Build history of the part. All positions in model axes, mm. A direction names the side the tool comes from. Give positions to 0.01 mm unless a question says otherwise; leave off trailing zeros. Order: outer loops, then holes, each group sorted by start corner. A loop starts at its lowest first (then second) coordinate and runs counter-clockwise, first axis right, second up. Notation, with made-up numbers: (-35, 81) - (19, 81) arc R11 cw to (19, 86) - close; hole circle Ø11 at (-39, 87.5). An arc over 180 degrees is marked (long way). Use a Markdown table: item, result. Add a question column.
(1) Slice it at A-A (z = 40). Write the cut outline in (x, y), then the cut area to 3 significant figures.
(2) Flat gauge pins, fed straight in: pin 1 (6 mm diameter, centred on x = -19, z = 55.5, fed in from -Y); pin 2 (9 mm diameter, centred on y = 9, z = 10, fed in from -X); pin 3 (0.6 mm diameter, centred on y = -11.5, z = 50, fed in from +X). Where does each tip first touch, or does it go through?
(3) Which spindle directions (+Z, -Z, +X, -X, +Y, -Y) get a long thin tool onto all of the face, cutting with end or side? Do faces 5 (the face through (-2.03, -33.32, 8.52)), 6 (the face through (-4, 11, 39)), 7 (the face through (-8, -22, 39)), 8 (the face through (-17, -26, 39)). Say none if no direction does.
(4) Slice it at B-B (z = 10). Write the cut outline in (x, y), then the cut area to 3 significant figures.
(5) Slice it at C-C (x = -14). Write the cut outline in (y, z), then the cut area to 3 significant figures.
(6) Wall check: line 1 (Y direction, x = -1.5, z = 70); line 2 (Z direction, x = -2.3, y = 9); line 3 (Z direction, x = -9, y = -24.9). Give the ranges that are in metal, low to high.
(7) Mould opens along Z. For faces 1 (the face through (-29, -11, 39)), 2 (the face through (-19, -22, 0)), 3 (the face through (-14, -24, 80)), 4 (the face through (-9.121, 2.028, 22.747)) say: +Z half, -Z half, draft (parallel to the pull), parting line (faces both ways), or undercut.
(8) Slice it at D-D (y = 9). Write the cut outline in (x, z).
Autodesk Inventor part; units mm, degrees
ref_plane "YZ Plane" through (0, 0, 0) normal (1, 0, 0) x (0, 1, 0)
ref_plane "XZ Plane" through (0, 0, 0) normal (0, 1, 0) x (-1, 0, 0)
ref_plane "XY Plane" through (0, 0, 0) normal (0, 0, 1) x (1, 0, 0)
sketch "Sketch1" plane through (0, 0, 0) normal (0, 0, 1) x (1, 0, 0)
  line L0 (0, 0) -> (-29, 0)
  line L1 (-29, 0) -> (-29, 4)
  line L2 (-29, 4) -> (-4, 4)
  line L3 (-4, 4) -> (-4, 18)
  line L4 (-4, 18) -> (0, 18)
  line L5 (0, 18) -> (0, 0)
  dimension "d0" = 4
  dimension "d1" = 4
  dimension "d2" = 29
  dimension "d3" = 18
extrude "Extrusion1" add sketch "Sketch1" along normal blind 80
sketch "Sketch3" plane through (0, 0, 0) normal (1, 0, 0) x (0, 0, -1)
  line L0 (0, 0) -> (-80, 0)
  line L1 (-80, 0) -> (-80, 18)
  line L2 (0, 0) -> (0, 18)
  point P0 (-70, 9)
  point P1 (-10, 9)
  dimension "d9" = 9
  dimension "d10" = 10
  dimension "d11" = 10
hole "Hole1" at (0, 9, 70) at (0, 9, 10) direction (-1, 0, 0) diameter 5.5 end through all
sketch "Sketch4" plane through (-29, 0, 0) normal (0, -1, 0) x (1, 0, 0)
  line L0 (29, 0) -> (29, 80)
  line L1 (0, 0) -> (29, 0)
  point P0 (20, 60)
  point P1 (20, 20)
  dimension "d19" = 9
  dimension "d20" = 20
  dimension "d21" = 20
hole "Hole2" at (-9, 0, 60) at (-9, 0, 20) direction (0, 1, 0) diameter 5.5 end through all
sketch "Sketch9" plane through (-29, 0, 0) normal (0, -1, 0) x (1, 0, 0)
  line L0 (25, 80) -> (0, 80)
  line L1 (25, 0) -> (0, 0)
  line L2 (0, 80) -> (3, 80)
  line L3 (3, 80) -> (3, 0)
  line L4 (3, 0) -> (0, 0)
  line L5 (0, 0) -> (0, 80)
  point P0 (29, 0)
  point P1 (3, 80)
  dimension "d57" = 3
extrude "Extrusion5" add sketch "Sketch9" along normal blind 26
sketch "Sketch10" plane through (-26, 0, 80) normal (1, 0, 0) x (0, 0, -1)
  line L0 (80, -26) -> (0, -26)
  line L1 (80, 4) -> (80, -26)
  line L2 (0, -26) -> (80, -26)
  line L3 (80, -26) -> (80, -22)
  line L4 (80, -22) -> (0, -22)
  line L5 (0, -22) -> (0, -26)
  point P0 (80, 0)
  dimension "d60" = 4
extrude "Extrusion6" add sketch "Sketch10" along normal blind 26
sketch "Sketch11" plane through (-29, -26, 0) normal (0, -1, 0) x (1, 0, 0)
  line L0 (29, 80) -> (25, 80)
  line L1 (25, 0) -> (0, 0)
  line L2 (29, 80) -> (25, 80)
  line L3 (25, 80) -> (25, 0)
  line L4 (25, 0) -> (29, 0)
  line L5 (29, 0) -> (29, 80)
  point P0 (29, 0)
  dimension "d63" = 4
extrude "Extrusion7" add sketch "Sketch11" along normal blind 14
sketch "Sketch12" plane through (0, 0, 80) normal (1, 0, 0) x (0, 0, -1)
  circle A0 centre (10, 9) radius 2.75
  circle A1 centre (70, 9) radius 2.75
  line L0 (80, 18) -> (0, 18)
  line L1 (80, -40) -> (0, -40)
  line L2 (80, -22) -> (0, -22)
  point P0 (80, 0)
  point P1 (10, -31)
  point P2 (70, -31)
  point P3 (51, 18)
  dimension "d66" = 9
  dimension "d85" = 9
hole "Hole5" at (0, -31, 70) at (0, -31, 10) direction (-1, 0, 0) diameter 5.5 end through all
sketch "Sketch14" plane through (-26, -22, 80) normal (0, 1, 0) x (1, 0, 0)
  circle A0 centre (17, 20) radius 2.75
  circle A1 centre (17, 60) radius 2.75
  point P0 (26, 80)
hole "Hole6" at (-9, -22, 60) at (-9, -22, 20) direction (0, -1, 0) diameter 5.5 end through all
sketch "Sketch24" plane through (0, 0, 80) normal (1, 0, 0) x (0, 0, -1)
  line L0 (80, -40) -> (0, -40)
  line L1 (0, -22) -> (0, -40)
  point P0 (80, 0)
  point P1 (40, -31.5)
  dimension "d157" = 8.5
  dimension "d158" = 40
hole "Hole9" at (0, -31.5, 40) direction (-1, 0, 0) diameter 4.5 depth 8 tip angle 118
fillet "Fillet1" radius 10 2 edges at (-26, -22, 40) (-26, 0, 40)
Solution:
| question | item | result |
|---|---|---|
| 1 | outline | (-29, -26) - (-4, -26) - (-4, -29.25) - (0, -29.25) - (0, -22) - (-16, -22) arc R10 cw to (-26, -12) - (-26, -10) arc R10 cw to (-16, 0) - (0, 0) - (0, 18) - (-4, 18) - (-4, 4) - (-29, 4) - close; (-4, -40) - (0, -40) - (0, -33.75) - (-4, -33.75) - close |
| 1 | area | 435 mm2 |
| 2 | pin 1 | y = -26 |
| 2 | pin 2 | x = -4 |
| 2 | pin 3 | x = -26 |
| 3 | face 5 | +X, -X |
| 3 | face 6 | +Z, -Z, -X, +Y |
| 3 | face 7 | +Z, -Z, +X |
| 3 | face 8 | +Z, -Z, -X, -Y |
| 4 | outline | (-29, -26) - (-4, -26) - (-4, -28.25) - (0, -28.25) - (0, -22) - (-16, -22) arc R10 cw to (-26, -12) - (-26, -10) arc R10 cw to (-16, 0) - (0, 0) - (0, 6.25) - (-4, 6.25) - (-4, 4) - (-29, 4) - close; (-4, -40) - (0, -40) - (0, -33.75) - (-4, -33.75) - close; (-4, 11.75) - (0, 11.75) - (0, 18) - (-4, 18) - close |
| 4 | area | 409 mm2 |
| 5 | outline | (-26, 0) - (-22, 0) - (-22, 80) - (-26, 80) - close; (0, 0) - (4, 0) - (4, 80) - (0, 80) - close |
| 5 | area | 640 mm2 |
| 6 | line 1 | -40 to -33.75, -28.25 to -22, 0 to 6.25, 11.75 to 18 |
| 6 | line 2 | 0 to 7.25, 12.75 to 67.25, 72.75 to 80 |
| 6 | line 3 | 0 to 17.25, 22.75 to 57.25, 62.75 to 80 |
| 7 | face 1 | draft |
| 7 | face 2 | -Z half |
| 7 | face 3 | +Z half |
| 7 | face 4 | undercut |
| 8 | outline | (-4, 0) - (0, 0) - (0, 7.25) - (-4, 7.25) - close; (-4, 12.75) - (0, 12.75) - (0, 67.25) - (-4, 67.25) - close; (-4, 72.75) - (0, 72.75) - (0, 80) - (-4, 80) - close |
